Study the drawing (mm; zero at the part's minimum x, y, z) and answer. A direction names the side the tool comes from. Coordinates: 2 decimals unless noted, no trailing zeros. Loops run counter-clockwise (first coordinate to the right, second up) from the corner with the lowest first, then second, coordinate; pieces in that order, holes last. Notation, with made-up numbers: M -28,19.25 L 16,19.25 A23 cw 16,47.25 Z; hole C 69.5,64.5 d8. An arc over 180 degrees is marked long. Use one line per item in the form item = value. Start each with the question number.
1. The part is cut by section B-B (y = 6.75). Give the vertices of the cut face in (x, z).
2. Flat-ended cylindrical pins translate along their axes: pin 1 (6 mm diameter, centred on x = 85, z = 21, fed in from -Y); pin 2 (1.5 mm diameter, centred on x = 39.5, z = 44.5, fed in from +Y); pin 3 (1.5 mm diameter, centred on x = 27, y = 5, fed in from -Z); pin 4 (1.5 mm diameter, centred on x = 83, y = 5.5, fed in from +Z). Find the tip coordinate at first contact, or state that the pin passes through.
3. The part is cut by section A-A (z = 25.5). Give the vertices of the cut face in (x, y), plus the area to 3 significant figures.
4. The part is cut by section C-C (x = 38). Give the vertices of the cut face in (y, z).
5. The part is cut by section D-D (y = 2). Give the vertices of the cut face in (x, z).
6. A tool of negligible diameter and unlimited length cuts with its end or side. For the marked faces 1, 2, 3, 4 and 5, from which of +Z, -Z, +X, -X, +Y, -Y can it reach the whole face along a straight path? Write none if from no direction.
7. Find the intervals of material crossed by probe 1 along X at (y, z) = (9.75, 35); probe 2 along Z at (x, y) = (26.5, 6.75); probe 3 along Y at (x, z) = (90, 40), in increasing order. Write a range as [from, to].
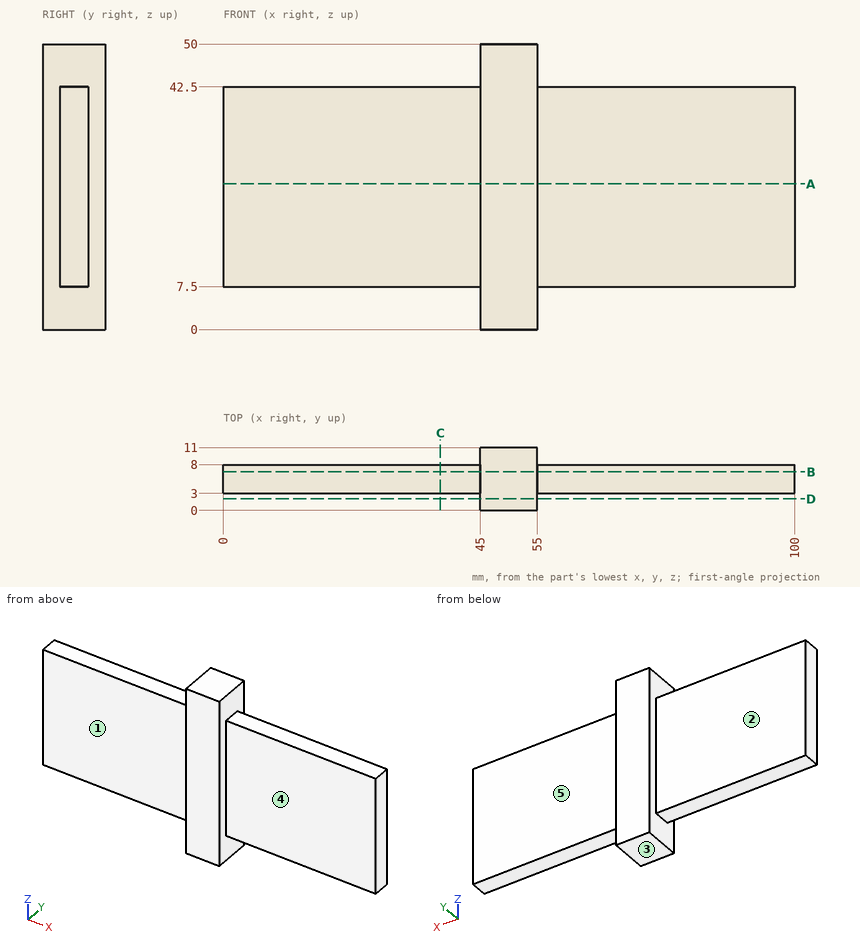
Computed values:
q1.outline = M 0,7.5 L 45,7.5 L 45,0 L 55,0 L 55,7.5 L 100,7.5 L 100,42.5 L 55,42.5 L 55,50 L 45,50 L 45,42.5 L 0,42.5 Z
q2.pin_1 = 3
q2.pin_2 = through
q2.pin_3 = 7.5
q2.pin_4 = 42.5
q3.outline = M 0,3 L 45,3 L 45,0 L 55,0 L 55,3 L 100,3 L 100,8 L 55,8 L 55,11 L 45,11 L 45,8 L 0,8 Z
q3.area = 560 mm²
q4.outline = M 3,7.5 L 8,7.5 L 8,42.5 L 3,42.5 Z
q5.outline = M 45,0 L 55,0 L 55,50 L 45,50 Z
q6.face_1 = +Z, -Z, -X, -Y
q6.face_2 = +Z, -Z, -X, +Y
q6.face_3 = -Z, +X, -X, +Y, -Y
q6.face_4 = +Z, -Z, +X, -Y
q6.face_5 = +Z, -Z, +X, +Y
q7.probe_1 = [45, 55]
q7.probe_2 = [7.5, 42.5]
q7.probe_3 = [3, 8]
